Can you work these out from the model? Positions are in its coordinate system, mm. A direction names the side the tool comes from. Round coordinates to 2 decimals unless told otherwise and drop trailing zeros. Loops run counter-clockwise (first coordinate to the right, second up) from the corner with the lowest first, then second, coordinate; pieces in that order, holes last. Notation, with made-up numbers: M 81,87.5 L 94,87.5 A23 ccw 94,96.5 Z; hole C 60.5,-8 d7. An arc over 180 degrees is marked long. Answer as CSV lines item,"result".
Autodesk Inventor part; units mm, degrees
ref_plane "YZ Plane" through (0, 0, 0) normal (1, 0, 0) x (0, 1, 0)
ref_plane "XZ Plane" through (0, 0, 0) normal (0, 1, 0) x (-1, 0, 0)
ref_plane "XY Plane" through (0, 0, 0) normal (0, 0, 1) x (1, 0, 0)
sketch "Sketch1" plane through (0, 0, 0) normal (1, 0, 0) x (0, 1, 0)
  line L0 (0, 18.823) -> (0, -81.823)
  line L1 (-50.323, 0) -> (13.573, 0)
  line L2 (0, 0) -> (0, -63)
  line L3 (0, -63) -> (-28, -63)
  line L4 (-28, -63) -> (-28, -24.33)
  line L5 (-28, -24.33) -> (-36.75, -24.33)
  line L6 (-36.75, -24.33) -> (-36.75, 0)
  line L7 (-36.75, 0) -> (0, 0)
  circle A0 centre (-16, -42.5) radius 1.575 construction
  line L8 (-35.988, -0.762) -> (-35.988, -23.568)
  line L9 (-35.988, -23.568) -> (-27.238, -23.568)
  line L10 (-27.238, -23.568) -> (-27.238, -62.238)
  line L11 (-27.238, -62.238) -> (-0.762, -62.238)
  line L12 (-0.762, -62.238) -> (-0.762, -0.762)
  line L13 (-0.762, -0.762) -> (-35.988, -0.762)
  line L14 (-41.195, 4.445) -> (-41.195, -28.775)
  line L15 (-41.195, -28.775) -> (-32.445, -28.775)
  line L16 (-32.445, -28.775) -> (-32.445, -67.445)
  line L17 (-32.445, -67.445) -> (4.445, -67.445)
  line L18 (4.445, -67.445) -> (4.445, 4.445)
  line L19 (4.445, 4.445) -> (-41.195, 4.445)
  line L20 (1.905, 1.905) -> (-29.905, 1.905) construction
  line L21 (-29.905, 1.905) -> (-29.905, -64.905) construction
  line L22 (-29.905, -64.905) -> (1.905, -64.905) construction
  line L23 (1.905, -64.905) -> (1.905, 1.905) construction
  line L24 (0.508, -63.508) -> (0.508, 0.508)
  line L25 (0.508, 0.508) -> (-37.258, 0.508)
  line L26 (-37.258, 0.508) -> (-37.258, -24.838)
  line L27 (-37.258, -24.838) -> (-28.508, -24.838)
  line L28 (-28.508, -24.838) -> (-28.508, -63.508)
  line L29 (-28.508, -63.508) -> (0.508, -63.508)
  dimension "d0" = 63
  dimension "d1" = 28
  dimension "d2" = 36.75
  dimension "d3" = 24.33
  dimension "d4" = 42.5
  dimension "d5" = 16
  dimension "d6" = 3.15
  dimension "d16" = 0.762
  dimension "d17" = 4.445
  dimension "d18" = 2.54
  dimension "d19" = 2.54
  dimension "d20" = 2.54
  dimension "d21" = 2.54
  dimension "d29" = 0.508
extrude "Extrusion1" add sketch "Sketch1" against normal blind 1.55 contours L25 L26 L1 L14 L19 L0 | L0 L19 L18 L1 L24 L25 | L1 L18 L17 L0 L29 L24 | L0 L17 L16 L15 L14 L1 L26 L27 L28 L29
hole "Hole1" at (0, -16, -42.5) direction (-1, 0, 0) diameter 3.15 end through all
hole "Hole2" at (0, 1.905, 1.905) at (0, -29.905, -64.905) direction (-1, 0, 0) diameter 2.6 end through all
equation "\"d20\" = d18"
equation "\"d21\" = d18"
properties part number "J010360" material "ACRYLIC, BLACK"
Item 1: If we section it at A-A on y = -0.5: Write out the boundary of the cut face in (x, z) (3 decimals), then the cut area to 3 significant figures.
Output:
outline,"M -1.55,-67.445 L 0,-67.445 L 0,-63.508 L -1.55,-63.508 Z; M -1.55,0.508 L 0,0.508 L 0,4.445 L -1.55,4.445 Z"
area,"12.2 mm2"
Item 2: If I drill on line 1 along Z through (x, y) = (-1.35, -33.5) (3 decimals); line 2 along Y through (x, z) = (-0.55, -21) (3 decimals); line 3 along Z through (x, y) = (-0.95, -14) (3 decimals), over which ranges is the centre line in solid material (lowest first)? Write a range as from..to.
Output:
line 1,"z = -28.775..-24.838, 0.508..4.445"
line 2,"y = -41.195..-37.258, 0.508..4.445"
line 3,"z = -67.445..-63.508, 0.508..4.445"
Item 3: If we section it at C-C on x = -1.2: Write out the boundary of the cut face in (y, z) (3 decimals).
Output:
outline,"M -41.195,-28.775 L -32.445,-28.775 L -32.445,-67.445 L 4.445,-67.445 L 4.445,4.445 L -41.195,4.445 Z; hole M -37.258,-24.838 L -28.508,-24.838 L -28.508,-63.508 L 0.508,-63.508 L 0.508,0.508 L -37.258,0.508 Z; hole C -29.905,-64.905 d2.6; hole C 1.905,1.905 d2.6"
Item 4: If we section it at B-B on z = -26.5: Write out the boundary of the cut face in (x, y) (3 decimals), then the cut area to 3 significant figures.
Output:
outline,"M -1.55,-41.195 L 0,-41.195 L 0,-28.508 L -1.55,-28.508 Z; M -1.55,0.508 L 0,0.508 L 0,4.445 L -1.55,4.445 Z"
area,"25.8 mm2"
Item 5: Will these pins go through, and if not, where does the flat tip stop? pin 1 (0.5 mm diameter, centred on x = -1, z = -57, fed in from -Y) (3 decimals); pin 2 (0.5 mm diameter, centred on x = -1, y = -36.5, fed in from -Z) (3 decimals).
Output:
pin 1,"stops at y = -32.445"
pin 2,"stops at z = -28.775"
Item 6: We'd pull the mould along Z, two halves only. Please class faces 4 (the face through (-1, -18, 4.445)), 5 (the face through (-1, -33, -24.838)), 6 (the face through (-1, -14, -67.445)): released by +Z, released by -Z, zero draft, split by the parting line, or undercut.
Output:
face 4,"released by +Z"
face 5,"undercut"
face 6,"released by -Z"
Item 7: On a 3-axis mill with a long thin cutter (end or side, diameter ignored), from which of +Z, -Z, +X, -X, +Y, -Y can I reach the whole of each face in a straight line? I mean faces 1 (the face through (-1, -32.445, -48)), 2 (the face through (0, -29, -29)), 3 (the face through (-1, -37.258, -12)). Say none if no direction works.
Output:
face 1,"-Z, +X, -X, -Y"
face 2,"+Z, -Z, +X, +Y, -Y"
face 3,"+X, -X"
